Check sheet for the modelled part. Datum: model origin and axes. Units: mm. A direction names the side the tool comes from. Round coordinates to 2 decimals unless told otherwise and drop trailing zeros. Order: outer loops, then holes, each group sorted by start corner. A loop starts at its lowest first (then second) coordinate and runs counter-clockwise, first axis right, second up. Notation, with made-up numbers: (-8.5, 38) -> (17.5, 38) arc R19 ccw to (17.5, 58) -> close; hole circle Ø5 at (34.25, 27). An arc over 180 degrees is marked (long way). Answer in a Markdown table with one row per item. Add a question column.
1. Sectioned sample at B-B, the plane z = 2.3. Record the boundary of the cut face in (x, y) (1 decimal).
2. Draft check along X on faces 1 (the flat face through (12.7, -18, 2)), 2 (the flat face through (7.73, -14.88, 0.78)), 3 (the cylindrical face through (0.178, -22.498, 0.382)). Enter one of: +X half, -X half, draft (parallel to the pull), parting line (faces both ways), or undercut.
3. Sectioned sample at D-D, the plane x = -0.5. Record the boundary of the cut face in (y, z) (1 decimal), then the cut area to 3 significant figures.
4. Access from +Z, -Z, +X, -X, +Y, -Y to the whole of each face (thin tool, end or side, straight path). Record for faces 4 (the cylindrical face through (-9.36, -18.62, 2.37)), 5 (the flat face through (-1.288, 14.356, 0.783)).
5. Sectioned sample at C-C, the plane y = 8.5. Record the boundary of the cut face in (x, z) (3 decimals).
6. Material ranges on L1, parallel to X at y = -17, z = 2.55; L2, parallel to X at y = -15, z = 0.8; L3, parallel to Y at x = -1, z = 0.15, recorded low to high. Write a range as from..to.
7. Sectioned sample at A-A, the plane x = 9.75. Record the boundary of the cut face in (y, z) (1 decimal).
8. Depth check by flat-ended pin: P1, Ø5, axis at x = 6, y = 5, coming from the +Z side (3 decimals); P2, Ø1.3, axis at y = 12, z = 1, coming from the +X side; P3, Ø4, axis at x = 9.02, y = -17.07, coming from the -Z side; P4, Ø1, axis at x = 9.5, z = 1, coming from the +Y side. Enter the tip coordinate at first touch or a pass-through.
```python
from build123d import *

# Parameters (mm, degrees)
F0_R     = 1.5875
F1_DEPTH = 3.175
F2_R     = 1.27
F4_DEPTH = 1.5875


with BuildPart() as f1:
    # F0 (on Top) → F1 (new body)
    with BuildSketch(Plane.XY):
        with BuildLine():
            ThreePointArc((0, 13.7541), (1.122532, 13.289132), (1.5875, 12.1666))
            ThreePointArc((1.5875, 12.1666), (1.122532, 11.044068), (0, 10.5791))
            Line((0, 10.5791), (0, -22.86))
            Line((0, -22.86), (12.7, -22.86))
            Line((12.7, -22.86), (12.7, -13.462))
            Line((12.7, -13.462), (3.81, -13.462))
            Line((3.81, -13.462), (3.81, 22.86))
            Line((3.81, 22.86), (0, 22.86))
            Line((0, 22.86), (0, 21.600245))
            Line((0, 21.600245), (3.175, 21.600245))
            Line((3.175, 21.600245), (3.175, 19.568245))
            Line((3.175, 19.568245), (0, 19.568245))
            Line((0, 19.568245), (0, 13.7541))
        make_face()
        with Locations((9.017, -17.0688)):
            Circle(F0_R, mode=Mode.SUBTRACT)
        with BuildLine():
            ThreePointArc((0, 10.5791), (-1.5875, 12.1666), (0, 13.7541))
            Line((0, 13.7541), (0, 19.568245))
            Line((0, 19.568245), (-3.175, 19.568245))
            Line((-3.175, 19.568245), (-3.175, 21.600245))
            Line((-3.175, 21.600245), (0, 21.600245))
            Line((0, 21.600245), (0, 22.86))
            Line((0, 22.86), (-3.81, 22.86))
            Line((-3.81, 22.86), (-3.81, -13.462))
            Line((-3.81, -13.462), (-12.7, -13.462))
            Line((-12.7, -13.462), (-12.7, -22.86))
            Line((-12.7, -22.86), (0, -22.86))
            Line((0, -22.86), (0, 10.5791))
        make_face()
        with Locations((-9.017, -17.0688)):
            Circle(F0_R, mode=Mode.SUBTRACT)
    extrude(amount=F1_DEPTH)

    # F2
    f2_edges = [f1.edges().sort_by_distance(p)[0] for p in [
        (0, -22.86, 0),
    ]]
    fillet(f2_edges, radius=F2_R)

    # F3 (on face) → F4 (cut)
    with BuildSketch(Plane(origin=(0, 0, 0), x_dir=(1, 0, 0), z_dir=(0, 0, -1))):
        Polygon((-6.477, 18.53527), (-9.017, 20.001739), (-11.557, 18.53527), (-11.557, 15.60233), (-9.017, 14.135861), (-6.477, 15.60233), align=None)
        Polygon((9.017, 20.001739), (6.477, 18.53527), (6.477, 15.60233), (9.017, 14.135861), (11.557, 15.60233), (11.557, 18.53527), align=None)
        Polygon((2.54, -10.70013), (0, -9.233661), (-2.54, -10.70013), (-2.54, -13.63307), (0, -15.099539), (2.54, -13.63307), align=None)
    extrude(amount=-F4_DEPTH, mode=Mode.SUBTRACT)


solid = f1.part
```
Answer key:
| question | item | result |
|---|---|---|
| 1 | outline | (-12.7, -22.9) -> (12.7, -22.9) -> (12.7, -13.5) -> (3.8, -13.5) -> (3.8, 22.9) -> (-3.8, 22.9) -> (-3.8, -13.5) -> (-12.7, -13.5) -> close; hole circle Ø3.2 at (-9, -17.1); hole (-3.2, 19.6) -> (3.2, 19.6) -> (3.2, 21.6) -> (-3.2, 21.6) -> close; hole circle Ø3.2 at (0, 12.2); hole circle Ø3.2 at (9, -17.1) |
| 2 | face 1 | +X half |
| 2 | face 2 | undercut |
| 2 | face 3 | draft |
| 3 | outline | (-22.9, 1.3) arc R1.3 ccw to (-21.6, 0) -> (9.5, 0) -> (9.5, 1.6) -> (10.7, 1.6) -> (10.7, 3.2) -> (-22.9, 3.2) -> close; (13.7, 1.6) -> (14.8, 1.6) -> (14.8, 0) -> (19.6, 0) -> (19.6, 3.2) -> (13.7, 3.2) -> close; (21.6, 0) -> (22.9, 0) -> (22.9, 3.2) -> (21.6, 3.2) -> close |
| 3 | area | 125 mm² |
| 4 | face 4 | +Z, -Z |
| 4 | face 5 | -Z |
| 5 | outline | (-3.81, 0) -> (3.81, 0) -> (3.81, 3.175) -> (-3.81, 3.175) -> close |
| 6 | L1 | x = -12.7..-10.6, -7.43..7.43, 10.6..12.7 |
| 6 | L2 | x = -12.7..-10.51, -7.52..7.52, 10.51..12.7 |
| 6 | L3 | y = -22.19..9.81, 14.52..19.57, 21.6..22.86 |
| 7 | outline | (-22.9, 1.3) arc R1.3 ccw to (-21.6, 0) -> (-19.6, 0) -> (-19.6, 1.6) -> (-18.5, 1.6) -> (-18.5, 3.2) -> (-22.9, 3.2) -> close; (-15.7, 1.6) -> (-14.6, 1.6) -> (-14.6, 0) -> (-13.5, 0) -> (-13.5, 3.2) -> (-15.7, 3.2) -> close |
| 8 | P1 | stops at z = 3.175 |
| 8 | P2 | stops at x = 3.81 |
| 8 | P3 | stops at z = 1.59 |
| 8 | P4 | stops at y = -13.46 |
